```python
from build123d import *

# Parameters (mm, degrees)
BOSS_EXTRUDE1_DEPTH = 3.175
SKETCH2_R           = 14.2875
CUT_EXTRUDE1_DEPTH  = 3.175


with BuildPart() as part:
    # Sketch1 → Boss-Extrude1 (new body)
    with BuildSketch(Plane.XY):
        Polygon((36.180133555, -50.152996979), (36.180133555, 19.697003021), (29.830133555, 83.197003021), (-1.919866445, 89.547003021), (-33.669866445, 83.197003021), (-40.019866445, 19.697003021), (-40.019866445, -50.152996979), align=None)
    extrude(amount=BOSS_EXTRUDE1_DEPTH)

    # Sketch2 → Cut-Extrude1 (cut)
    with BuildSketch(Plane.XY.offset(3.175)):
        with Locations((-1.919866445, 47.205203021)):
            Circle(SKETCH2_R)
    extrude(amount=-CUT_EXTRUDE1_DEPTH, mode=Mode.SUBTRACT)


solid = part.part
```
Could you check a few things on this model? Use its own coordinates, in mm. Round coordinates to 2 decimals unless told otherwise and drop trailing zeros. Loops run counter-clockwise (first coordinate to the right, second up) from the corner with the lowest first, then second, coordinate; pieces in that order, holes last. Notation, with made-up numbers: M -6,-15.75 L 1,-15.75 A15 ccw 1,3.25 Z; hole C -15,36.5 d9. An arc over 180 degrees is marked long. Put each result on its own line as item: value.
Q1. Imagine slicing it at A-A (x = 5.5). Write out the boundary of the cut face in (y, z) (3 decimals), then the cut area to 3 significant figures.
Check result:
outline: M -50.153,0 L 34.995,0 L 34.995,3.175 L -50.153,3.175 Z; M 59.415,0 L 88.063,0 L 88.063,3.175 L 59.415,3.175 Z
area: 361 mm2
Q2. Thinking about a two-plate mould opening in Y: for faces 1 (the face through (-3.78, 61.37, 1.61)), 2 (the face through (33.05, 51, 1.57)), 3 (the face through (-2, -50.153, 2)), which applies, released by +Y, released by -Y, zero draft, split by the parting line, or undercut?
Check result:
face 1: undercut
face 2: released by +Y
face 3: released by -Y
Q3. I need wall thicknesses on probe 1 along Y at (x, z) = (-10, 2.35); probe 2 along Y at (x, z) = (-5.5, 2.65); probe 3 along X at (y, z) = (41, 0.9). Which ranges of each line are inside material? Lowest first, please.
Check result:
probe 1: -50.15 to 35.42, 58.99 to 87.93
probe 2: -50.15 to 33.37, 61.04 to 88.83
probe 3: -37.89 to -14.79, 10.95 to 34.05
Q4. For pin 1 (1.5 mm diameter, centred on y = 71, z = 0.5, fed in from -X), with a flat end and sliding along its axis, tell me the tip position at first contact or that it passes through.
Check result:
pin 1: x = -34.96
Q5. Imagine slicing it at C-C (z = 1.85). Write out the boundary of the cut face in (x, y) (1 decimal).
Check result:
outline: M -40,-50.2 L 36.2,-50.2 L 36.2,19.7 L 29.8,83.2 L -1.9,89.5 L -33.7,83.2 L -40,19.7 Z; hole C -1.9,47.2 d28.6
Q6. Imagine slicing it at D-D (x = 27.5). Write out the boundary of the cut face in (y, z) (3 decimals).
Check result:
outline: M -50.153,0 L 83.663,0 L 83.663,3.175 L -50.153,3.175 Z
Q7. Imagine slicing it at B-B (y = 57.5). Write out the boundary of the cut face in (x, z) (3 decimals), then the cut area to 3 significant figures.
Check result:
outline: M -36.24,0 L -11.827,0 L -11.827,3.175 L -36.24,3.175 Z; M 7.987,0 L 32.4,0 L 32.4,3.175 L 7.987,3.175 Z
area: 155 mm2
